Design review of the part built by this model. Coordinates are the model's own, in mm. Face numbers are marked on the shaded views. A direction names the side the tool comes from. Coordinates: 2 decimals unless noted, no trailing zeros. Order: outer loops, then holes, each group sorted by start corner. A loop starts at its lowest first (then second) coordinate and runs counter-clockwise, first axis right, second up. Notation, with made-up numbers: (-19.5, 72) - (27.5, 72) arc R31 cw to (27.5, 97) - close; hole circle Ø8 at (8.25, 42). An arc over 180 degrees is marked (long way). Write each question's results on one line, items separated by ' | '. Start each with the question number.
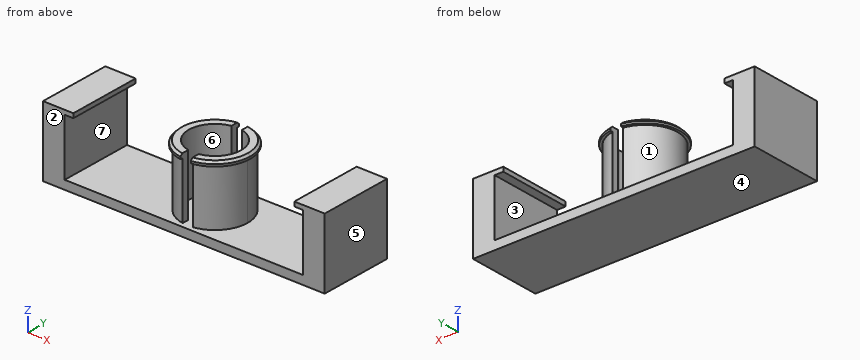
```python
from build123d import *

# Parameters (mm, degrees)
F1_DEPTH = 1
F2_W     = 2.5
F2_H     = 8.5
F3_DEPTH = 8
F5_W     = 1
F5_H     = 8.5
F6_DEPTH = 0.5
F9_DEPTH = 9
F10_SIZE = 0.25


with BuildPart() as f1:
    # F0 (on Top) → F1 (new body)
    with BuildSketch(Plane.XY):
        with BuildLine():
            Line((0, 8.5), (0, 0))
            Line((0, 0), (13.75, 0))
            Line((13.75, 0), (13.75, 0.5))
            ThreePointArc((13.75, 0.5), (10, 4.25), (13.75, 8))
            Line((13.75, 8), (13.75, 8.5))
            Line((13.75, 8.5), (0, 8.5))
        make_face()
        with BuildLine():
            Line((13.75, 0.5), (13.75, 0))
            Line((13.75, 0), (27.5, 0))
            Line((27.5, 0), (27.5, 8.5))
            Line((27.5, 8.5), (13.75, 8.5))
            Line((13.75, 8.5), (13.75, 8))
            ThreePointArc((13.75, 8), (16.4016504294, 6.9016504294), (17.5, 4.25))
            ThreePointArc((17.5, 4.25), (16.4016504294, 1.5983495706), (13.75, 0.5))
        make_face()
        with BuildLine():
            ThreePointArc((13.75, 8), (10, 4.25), (13.75, 0.5))
            Line((13.75, 0.5), (13.75, 8))
        make_face()
        with BuildLine():
            Line((13.75, 8), (13.75, 0.5))
            ThreePointArc((13.75, 0.5), (16.4016504294, 1.5983495706), (17.5, 4.25))
            ThreePointArc((17.5, 4.25), (16.4016504294, 6.9016504294), (13.75, 8))
        make_face()
    extrude(amount=F1_DEPTH)

    # F2 (on Top) → F3 (join)
    with BuildSketch(Plane.XY):
        with Locations((-1.25, 4.25)):
            Rectangle(F2_W, F2_H)
        with BuildLine():
            ThreePointArc((13.75, 8), (10, 4.25), (13.75, 0.5))
            Line((13.75, 0.5), (13.75, 8))
        make_face()
        with BuildLine():
            Line((13.75, 8), (13.75, 0.5))
            ThreePointArc((13.75, 0.5), (16.4016504294, 1.5983495706), (17.5, 4.25))
            ThreePointArc((17.5, 4.25), (16.4016504294, 6.9016504294), (13.75, 8))
        make_face()
        with Locations((28.75, 4.25)):
            Rectangle(F2_W, F2_H)
    extrude(amount=F3_DEPTH)

    # F5 (on offset) → F6 (join)
    with BuildSketch(Plane.XY.offset(8)):
        with Locations((27, 4.25)):
            Rectangle(F5_W, F5_H)
        with Locations((0.5, 4.25)):
            Rectangle(F5_W, F5_H)
        with BuildLine():
            ThreePointArc((13.75, 8.3), (9.7, 4.25), (13.75, 0.2))
            Line((13.75, 0.2), (13.75, 8.3))
        make_face()
        with BuildLine():
            Line((13.75, 8.3), (13.75, 0.2))
            ThreePointArc((13.75, 0.2), (16.6137824638, 1.3862175362), (17.8, 4.25))
            ThreePointArc((17.8, 4.25), (16.6137824638, 7.1137824638), (13.75, 8.3))
        make_face()
    extrude(amount=-F6_DEPTH)

    # F8 (on offset) → F9 (cut)
    with BuildSketch(Plane.XY.offset(10)):
        with BuildLine():
            Line((13.75, 1.25), (13.75, 0))
            Line((13.75, 0), (14.35, 0))
            Line((14.35, 0), (14.35, 1.3106123087))
            ThreePointArc((14.35, 1.3106123087), (14.051526886, 1.265191541), (13.75, 1.25))
        make_face()
        with BuildLine():
            Line((13.75, 8.5), (13.75, 7.25))
            ThreePointArc((13.75, 7.25), (14.051526886, 7.234808459), (14.35, 7.1893876913))
            Line((14.35, 7.1893876913), (14.35, 8.5))
            Line((14.35, 8.5), (13.75, 8.5))
        make_face()
        with BuildLine():
            Line((13.75, 4.25), (13.75, 1.25))
            ThreePointArc((13.75, 1.25), (14.051526886, 1.265191541), (14.35, 1.3106123087))
            Line((14.35, 1.3106123087), (14.35, 4.25))
            Line((14.35, 4.25), (13.75, 4.25))
        make_face()
        with BuildLine():
            ThreePointArc((13.15, 7.1893876913), (10.75, 4.25), (13.15, 1.3106123087))
            Line((13.15, 1.3106123087), (13.15, 4.25))
            Line((13.15, 4.25), (13.15, 7.1893876913))
        make_face()
        with BuildLine():
            Line((13.15, 8.5), (13.15, 7.1893876913))
            ThreePointArc((13.15, 7.1893876913), (13.448473114, 7.234808459), (13.75, 7.25))
            Line((13.75, 7.25), (13.75, 8.5))
            Line((13.75, 8.5), (13.15, 8.5))
        make_face()
        with BuildLine():
            Line((13.75, 7.25), (13.75, 4.25))
            Line((13.75, 4.25), (14.35, 4.25))
            Line((14.35, 4.25), (14.35, 7.1893876913))
            ThreePointArc((14.35, 7.1893876913), (14.051526886, 7.234808459), (13.75, 7.25))
        make_face()
        with BuildLine():
            Line((13.15, 1.3106123087), (13.15, 0))
            Line((13.15, 0), (13.75, 0))
            Line((13.75, 0), (13.75, 1.25))
            ThreePointArc((13.75, 1.25), (13.448473114, 1.265191541), (13.15, 1.3106123087))
        make_face()
        with BuildLine():
            Line((14.35, 4.25), (14.35, 1.3106123087))
            ThreePointArc((14.35, 1.3106123087), (16.0737900077, 2.3526334039), (16.75, 4.25))
            ThreePointArc((16.75, 4.25), (16.0737900077, 6.1473665961), (14.35, 7.1893876913))
            Line((14.35, 7.1893876913), (14.35, 4.25))
        make_face()
        with BuildLine():
            Line((13.15, 4.25), (13.15, 1.3106123087))
            ThreePointArc((13.15, 1.3106123087), (13.448473114, 1.265191541), (13.75, 1.25))
            Line((13.75, 1.25), (13.75, 4.25))
            Line((13.75, 4.25), (13.75, 7.25))
            ThreePointArc((13.75, 7.25), (13.448473114, 7.234808459), (13.15, 7.1893876913))
            Line((13.15, 7.1893876913), (13.15, 4.25))
        make_face()
    extrude(amount=-F9_DEPTH, mode=Mode.SUBTRACT)

    # F10
    f10_edges = [f1.edges().sort_by_distance(p)[0] for p in [
        (9.7, 4.25, 8),
        (17.8, 4.25, 8),
    ]]
    chamfer(f10_edges, length=F10_SIZE)


solid = f1.part
```
(1) To check wall thickness, follow line 1 along X through (y, z) = (3.25, 6.75); line 2 along X through (y, z) = (8.25, 5); line 3 along X through (y, z) = (4.5, 2). State the ranges of each line that lie inside material, in increasing order. Write a range as [from, to].
(2) Take a section at A-A (z = 6.5). State the section outline as (x, y) points.
(3) Tool access review of the marked faces 5, 6 and 7: name each direction out of +Z, -Z, +X, -X, +Y, -Y from which nothing blocks a thin tool from reaching the whole face with its end or side.
(4) Mouldability with a two-part tool opening along Z and no side actions: class the marked faces 1, 2, 3 and 4 as +Z half, -Z half, draft (parallel to the pull), parting line (faces both ways), or undercut.
(5) Clearance check with flat-ended pins moving along their axes: pin 1 (1.5 mm diameter, centred on x = 13, z = 7, fed in from -Y); pin 2 (4 mm diameter, centred on x = 23.5, z = 3.5, fed in from +Y). State where each tip first meets the part, or that it passes through.
(6) Take a section at B-B (x = 2). State the section outline as (y, z) points.
Worked out:
1) line 1: [-2.5, 0], [10.14, 10.92], [16.58, 17.36], [27.5, 30] | line 2: [-2.5, 0], [27.5, 30] | line 3: [-2.5, 0], [10.01, 10.76], [16.74, 17.49], [27.5, 30]
2) outline: (-2.5, 0) - (0, 0) - (0, 8.5) - (-2.5, 8.5) - close; (13.15, 0.55) - (13.15, 1.31) arc R3 cw to (13.15, 7.19) - (13.15, 7.95) arc R3.75 ccw to start; (14.35, 0.55) arc R3.75 ccw to (14.35, 7.95) - (14.35, 7.19) arc R3 cw to (14.35, 1.31) - close; (27.5, 0) - (30, 0) - (30, 8.5) - (27.5, 8.5) - close
3) face 5: +Z, -Z, +X, +Y, -Y | face 6: +Z | face 7: +Y, -Y
4) face 1: undercut | face 2: draft | face 3: undercut | face 4: -Z half
5) pin 1: y = 0.24 | pin 2: through
6) outline: (0, 0) - (8.5, 0) - (8.5, 1) - (0, 1) - close
